from build123d import *

# Parameters (mm, degrees)
PAD_DEPTH         = 20
SKETCH002_R       = 21.818264
PAD001_DEPTH      = 30
POCKET_DEPTH      = 0.001
POCKET_DEPTH_BACK = -30.001
POCKET001_DEPTH   = 7
SKETCH005_R       = 5.295073
POCKET002_DEPTH   = 13.001
POCKET003_DEPTH   = 20.001


with BuildPart() as part:
    # Sketch001 → Pad (new body)
    with BuildSketch(Plane.XY):
        with BuildLine():
            ThreePointArc((13.179717, -17.387688), (21.818264, 0), (13.179717, 17.387688))
            Line((13.179717, 17.387688), (92.096497, 17.387688))
            Line((92.096497, 17.387688), (92.096497, -17.387688))
            Line((92.096497, -17.387688), (13.179717, -17.387688))
        make_face()
    extrude(amount=PAD_DEPTH)

    # Sketch002 → Pad001 (join)
    with BuildSketch(Plane.XY):
        Circle(SKETCH002_R)
    extrude(amount=PAD001_DEPTH)

    # Sketch003 → Pocket (cut, two sides)
    with BuildSketch(Plane.XY) as pocket_sk:
        with BuildLine():
            ThreePointArc((-10.409979, -5.074877), (11.581107, 0), (-10.409979, 5.074877))
            Line((-10.409979, 5.074877), (-15.391012, 5.074877))
            Line((-15.391012, 5.074877), (-15.391012, -5.074877))
            Line((-15.391012, -5.074877), (-10.409979, -5.074877))
        make_face()
    extrude(amount=-POCKET_DEPTH, mode=Mode.SUBTRACT)
    extrude(pocket_sk.sketch, amount=-POCKET_DEPTH_BACK, mode=Mode.SUBTRACT)

    # Sketch004 → Pocket001 (cut)
    with BuildSketch(Plane.XY.offset(20)):
        with BuildLine():
            ThreePointArc((25.04314, -8.428525), (26.423454, 0), (25.04314, 8.428525))
            ThreePointArc((28.188104, 12.650604), (25.510048, 11.36309), (25.04314, 8.428525))
            Line((74.586278, 12.650604), (28.188104, 12.650604))
            Line((74.586278, -12.650604), (74.586278, 12.650604))
            Line((28.188104, -12.650604), (74.586278, -12.650604))
            ThreePointArc((25.04314, -8.428525), (25.510048, -11.36309), (28.188104, -12.650604))
        make_face()
    extrude(amount=-POCKET001_DEPTH, mode=Mode.SUBTRACT)

    # Sketch005 (on Face18 of Pocket001) → Pocket002 (cut, through all)
    with BuildSketch(Plane.XY.offset(13)):
        with Locations((57.961857, 0)):
            Circle(SKETCH005_R)
        with Locations((38.617462, 0)):
            Circle(SKETCH005_R)
    extrude(amount=-POCKET002_DEPTH, mode=Mode.SUBTRACT)

    # Sketch006 (on Face5 of Pocket002) → Pocket003 (cut, through all)
    with BuildSketch(Plane.XY.offset(20)):
        Polygon((38.599522, 0), (38.599522, -29.031481), (99.493477, -29.031481), (99.493477, 19.057034), (72.520317, 19.057034), (72.520317, 0), align=None)
    extrude(amount=-POCKET003_DEPTH, mode=Mode.SUBTRACT)


solid = part.part
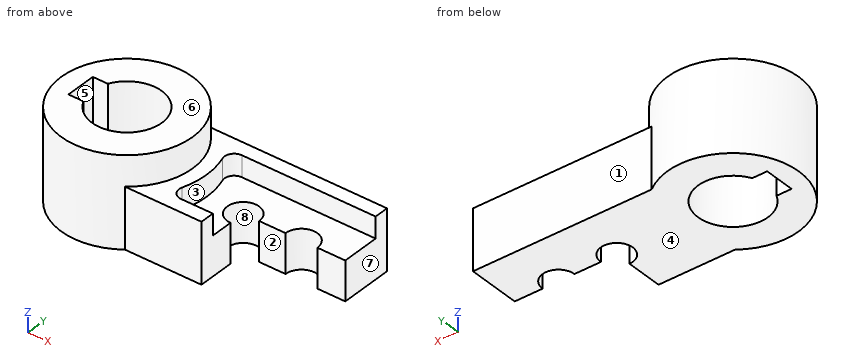
Work out the finished part from the listing and answer in its coordinate system (mm). Face numbers are marked on the shaded views. A direction names the side the tool comes from. Coordinates: 2 decimals unless noted, no trailing zeros. Write each loop counter-clockwise with the first axis right and the second up, starting at its lowest first coordinate (ties: lowest second). Pieces come first, ordered by that corner, then holes. Notation, with made-up numbers: M 4,80.5 L 54,80.5 A18 cw 54,92.5 Z; hole C -29,1.25 d1. An arc over 180 degrees is marked long. Write item = value, one per line.
1. Flat-ended cylindrical pins translate along their axes: pin 1 (1.5 mm diameter, centred on y = -7.5, z = 26, fed in from -X); pin 2 (4.5 mm diameter, centred on x = 50, z = 6.5, fed in from -Y); pin 3 (6 mm diameter, centred on y = -13, z = 13, fed in from +X); pin 4 (17 mm diameter, centred on x = 38.62, y = 0, fed in from -Z). Find the tip coordinate at first contact, or state that the pin passes through.
Solution:
pin_1 = -20.75
pin_2 = 0
pin_3 = 38.6
pin_4 = 0
2. Straight lines are drawn through the part: line 1 (Y direction, x = 0, z = 10.5); line 2 (Z direction, x = 19.5, y = 12); line 3 (Z direction, x = 30.5, y = -12). For each, find the intervals that lie inside material, in ascending order. Write a range as from..to.
Solution:
line_1 = -21.82..-11.58, 11.58..21.82
line_2 = 0..20
line_3 = 0..13
3. The part is cut by section B-B (z = 3). Determine the outline of the cut face in (x, y), then the cut area to 3 significant figures.
Solution:
outline = M 13.18,-17.39 L 38.6,-17.39 L 38.6,-5.3 A5.3 cw long 43.91,0 L 52.67,0 A5.3 cw 63.26,0 L 72.52,0 L 72.52,17.39 L 13.18,17.39 A21.82 ccw long Z; hole M -15.39,-5.07 L -10.41,-5.07 A11.58 ccw long -10.41,5.07 L -15.39,5.07 Z
area = 2,190 mm2
4. Determine the mould class of the marked faces 6, 7 and 8 for opening direction X: released by +X, released by -X, zero draft, split by the parting line, or undercut.
Solution:
face_6 = zero draft
face_7 = released by +X
face_8 = undercut
5. For the marked faces 1, 2, 3, 4 and 5, determine the directions among +Z, -Z, +X, -X, +Y, -Y from which every point of the face is accessible in a straight line to the end or side of a thin tool.
Solution:
face_1 = +Z, -Z, +X, +Y
face_2 = +Z, -Z, +X, -Y
face_3 = +Z, +X
face_4 = -Z, +X, -X, +Y, -Y
face_5 = +Z, -Z
6. The part is cut by section D-D (z = 21). Determine the outline of the cut face in (x, y), then the cut area to 3 significant figures.
Solution:
outline = C 0,0 d43.64; hole M -15.39,-5.07 L -10.41,-5.07 A11.58 ccw long -10.41,5.07 L -15.39,5.07 Z
area = 1,030 mm2
7. The part is cut by section C-C (x = 31). Determine the outline of the cut face in (y, z).
Solution:
outline = M -17.39,0 L 17.39,0 L 17.39,20 L 12.65,20 L 12.65,13 L -12.65,13 L -12.65,20 L -17.39,20 Z
8. The part is cut by section A-A (x = 0). Determine the outline of the cut face in (y, z), then the cut area to 3 significant figures.
Solution:
outline = M -21.82,0 L -11.58,0 L -11.58,30 L -21.82,30 Z; M 11.58,0 L 21.82,0 L 21.82,30 L 11.58,30 Z
area = 614 mm2
